Geometry: final body of the model. Coordinates: model frame, mm. Face numbers are marked on the shaded views. A direction names the side the tool comes from. Give positions to 0.01 mm unless a question says otherwise; leave off trailing zeros. Loops run counter-clockwise (first coordinate to the right, second up) from the corner with the lowest first, then second, coordinate; pieces in that order, holes last.
from build123d import *

# Parameters (mm, degrees)
BOSS_EXTRUDE1_DEPTH = 3.175
CUT_EXTRUDE1_REACH  = 105.449
SKETCH2_R           = 1.27
CUT_EXTRUDE2_DEPTH  = 104.449433541
FILLET1_R           = 10
FILLET2_R           = 0.25
FILLET3_R           = 3
FILLET4_R           = 0.5
FILLET5_R           = 7
FILLET6_R           = 3


with BuildPart() as part:
    # Sketch1 → Boss-Extrude1 (new body)
    with BuildSketch(Plane(origin=(0, 0, 0), x_dir=(1, 0, 0), z_dir=(0, 1, 0))):
        with BuildLine():
            Line((-30, 0), (-70, 0))
            Line((-70, 0), (-95.810939636, -36.861841993))
            ThreePointArc((-95.810939636, -36.861841993), (-95.670834686, -38.169513139), (-94.356227321, -38.207469686))
            Line((-94.356227321, -38.207469686), (-71.194689629, -19.140661569))
            Line((-71.194689629, -19.140661569), (-46.31139823, -21.55350411))
            ThreePointArc((-46.31139823, -21.55350411), (-45.254748427, -20.8377054), (-45.762041851, -19.666582016))
            Line((-45.762041851, -19.666582016), (-64.794329494, -10))
            Line((-64.794329494, -10), (-10, -10))
            Line((-10, -10), (-10, -15))
            ThreePointArc((-10, -15), (-5, -20), (0, -15))
            Line((0, -15), (0, 0))
            Line((0, 0), (-15, 0))
            Line((-15, 0), (-15, 13))
            ThreePointArc((-15, 13), (-15.585786438, 14.414213562), (-17, 15))
            Line((-17, 15), (-18.929632483, 15))
            ThreePointArc((-18.929632483, 15), (-19.873348334, 14.763349198), (-20.593733072, 14.109400392))
            Line((-20.593733072, 14.109400392), (-30, 0))
        make_face()
    extrude(amount=BOSS_EXTRUDE1_DEPTH)

    # Sketch2 → Cut-Extrude1 (cut, up to next)
    with BuildSketch(Plane(origin=(0, 3.175, 0), x_dir=(1, 0, 0), z_dir=(0, 1, 0)), mode=Mode.PRIVATE) as cut_extrude1_sk1:
        with Locations(Location((-5, -15, 0), (0, 0, 270))):
            Circle(SKETCH2_R)
    cut_extrude1_tool1 = extrude(cut_extrude1_sk1.sketch, amount=-CUT_EXTRUDE1_REACH, mode=Mode.PRIVATE) & part.part
    # Sketch2 → Cut-Extrude1 (cut, up to next)
    with BuildSketch(Plane(origin=(0, 3.175, 0), x_dir=(1, 0, 0), z_dir=(0, 1, 0)), mode=Mode.PRIVATE) as cut_extrude1_sk2:
        with Locations(Location((-17.964816242, 12, 0), (0, 0, 270))):
            Circle(SKETCH2_R)
    cut_extrude1_tool2 = extrude(cut_extrude1_sk2.sketch, amount=-CUT_EXTRUDE1_REACH, mode=Mode.PRIVATE) & part.part
    add(cut_extrude1_tool1.solids().sort_by_distance((-5, 3.175, 15))[0], mode=Mode.SUBTRACT)
    add(cut_extrude1_tool2.solids().sort_by_distance((-17.964816, 3.175, -12))[0], mode=Mode.SUBTRACT)

    # Sketch3 → Cut-Extrude2 (cut, through all)
    with BuildSketch(Plane(origin=(0, 3.175, 0), x_dir=(1, 0, 0), z_dir=(0, 1, 0))):
        with BuildLine():
            Line((-44, 0), (-40, 0))
            ThreePointArc((-40, 0), (-42, -2), (-44, 0))
        make_face()
    extrude(amount=-CUT_EXTRUDE2_DEPTH, mode=Mode.SUBTRACT)

    # Fillet1
    fillet1_edges = [part.edges().sort_by_distance(p)[0] for p in [
        (-70, 1.5875, 0),
    ]]
    fillet(fillet1_edges, radius=FILLET1_R)

    # Fillet2
    fillet2_edges = [part.edges().sort_by_distance(p)[0] for p in [
        (-64.794329494, 1.5875, 10),
    ]]
    fillet(fillet2_edges, radius=FILLET2_R)

    # Fillet3
    fillet3_edges = [part.edges().sort_by_distance(p)[0] for p in [
        (-10, 1.5875, 10),
    ]]
    fillet(fillet3_edges, radius=FILLET3_R)

    # Fillet4
    fillet4_edges = [part.edges().sort_by_distance(p)[0] for p in [
        (-40, 1.5875, 0),
        (-44, 1.5875, 0),
    ]]
    fillet(fillet4_edges, radius=FILLET4_R)

    # Fillet5
    fillet5_edges = [part.edges().sort_by_distance(p)[0] for p in [
        (0, 1.5875, 0),
    ]]
    fillet(fillet5_edges, radius=FILLET5_R)

    # Fillet6
    fillet6_edges = [part.edges().sort_by_distance(p)[0] for p in [
        (-15, 1.5875, 0),
    ]]
    fillet(fillet6_edges, radius=FILLET6_R)


solid = part.part
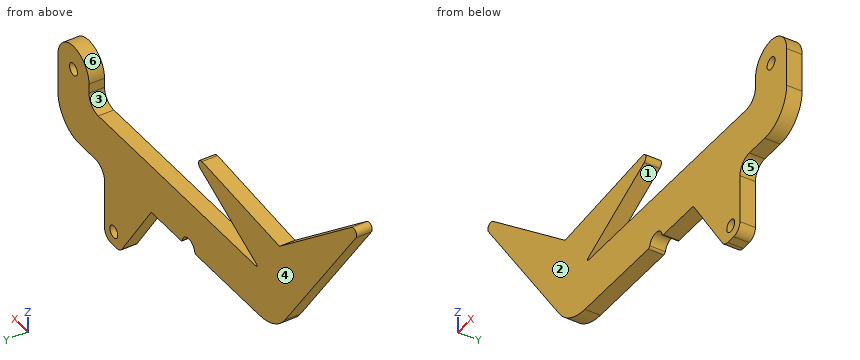
Item 1: Set-up query: the marked faces 1, 2 and 3. Return all of +Z, -Z, +X, -X, +Y, -Y with unobstructed straight access to the full face (end or side cutting, diameter ignored); none if empty.
Values follow:
face 1: +Y, -Y
face 2: +Z, -Z, +X, -X, -Y
face 3: +Z, +Y, -Y
Item 2: Section query A-A on z = -12. Return loops of the section in (x, y) (3 decimals), plus the area to 3 significant figures.
Values follow:
outline: (-22, 0) - (-19.235, 0) - (-19.235, 3.175) - (-22, 3.175) - close; (-16.695, 0) - (-15, 0) - (-15, 3.175) - (-16.695, 3.175) - close
area: 14.2 mm2
Item 3: Draft query along X for the marked faces 4, 5 and 6. Return one class per face: +X half, -X half, draft (parallel to the pull), parting line (faces both ways), or undercut.
Values follow:
face 4: draft
face 5: +X half
face 6: undercut
Item 4: Pin query (flat end, axial travel): pin 1 (1.6 mm diameter, centred on y = 2, z = -10.5, fed in from +X); pin 2 (1 mm diameter, centred on x = -33, y = 2, fed in from -Z); pin 3 (1.5 mm diameter, centred on y = 1, z = 26, fed in from -X). Return the tip coordinate at first contact, or that it passes through.
Values follow:
pin 1: stops at x = -15
pin 2: stops at z = 0
pin 3: stops at x = -88.73
Item 5: Section query B-B on x = -57.5. Return loops of the section in (y, z) (3 decimals).
Values follow:
outline: (0, 0) - (3.175, 0) - (3.175, 10) - (0, 10) - close; (0, 13.705) - (3.175, 13.705) - (3.175, 20.469) - (0, 20.469) - close
Item 6: Ray query, probe 1 along X at (y, z) = (2.25, 15); probe 2 along X at (y, z) = (2.15, -12); probe 3 along X at (y, z) = (0.5, 14.5). Return the intervals inside material, ascending.
Values follow:
probe 1: x = -80.5 to -54.95, -10 to -6.27, -3.73 to 0
probe 2: x = -22 to -19.23, -16.69 to -15
probe 3: x = -80.15 to -55.93, -10 to -6.17, -3.83 to 0
Item 7: Section query C-C on y = 1.15. Return loops of the section in (x, z).
Values follow:
outline: (-95.81, 36.86) - (-72.99, 4.26) arc R10 ccw to (-64.79, 0) - (-44.45, 0) arc R0.5 ccw to (-43.96, 0.4) arc R2 cw to (-40.04, 0.4) arc R0.5 ccw to (-39.55, 0) - (-30, 0) - (-20.59, -14.11) arc R2 ccw to (-18.93, -15) - (-17, -15) arc R2 ccw to (-15, -13) - (-15, -3) arc R3 cw to (-12, 0) - (-7, 0) arc R7 ccw to (0, 7) - (0, 15) arc R5 ccw to (-10, 15) - (-10, 13) arc R3 cw to (-13, 10) - (-63.75, 10) arc R0.25 cw to (-63.86, 10.47) - (-45.76, 19.67) arc R1 ccw to (-46.31, 21.55) - (-71.19, 19.14) - (-94.36, 38.21) arc R1 ccw to start; hole circle Ø2.54 at (-17.96, -12); hole circle Ø2.54 at (-5, 15)
Item 8: Section query D-D on x = -25. Return loops of the section in (y, z) (3 decimals), plus the area to 3 significant figures.
Values follow:
outline: (0, -7.5) - (3.175, -7.5) - (3.175, 10) - (0, 10) - close
area: 55.6 mm2
